Check sheet for the modelled part. Datum: model origin and axes. Units: mm. A direction names the side the tool comes from. Give positions to 0.01 mm unless a question says otherwise; leave off trailing zeros. Order: outer loops, then holes, each group sorted by start corner. A loop starts at its lowest first (then second) coordinate and runs counter-clockwise, first axis right, second up.
Item 1: Sectioned sample at D-D on x = 55.5. Record the boundary of the cut face in (y, z), and give its area (3 significant figures).
Item 2: Release check for a two-part mould opening along Y. For faces 1 (the flat face through (37.99, 15.8, 0.02)), 2 (the cylindrical face through (74.421, 46.854, 0.021)), 3 (the cylindrical face through (0, -20, 0)) record: released by +Y, released by -Y, zero draft, split by the parting line, or undercut.
Item 3: Sectioned sample at B-B on y = 0. Record the boundary of the cut face in (x, z), and give its area (3 significant figures).
Item 4: Sectioned sample at A-A on x = 0. Record the boundary of the cut face in (y, z).
Item 5: Material ranges on line 1 along X through (y, z) = (31.5, -0.2) (3 decimals); line 2 along X through (y, z) = (28.5, -0.85); line 3 along Y through (x, z) = (-65, -0.4) (3 decimals), recorded low to high.
Item 6: Sectioned sample at C-C on z = -1.05. Count the separate pieces of the cut face and the enclosed holes in it, and give its area (3 significant figures).
Item 7: Access from +Z, -Z, +X, -X, +Y, -Y to the whole of each face (thin tool, end or side, straight path). Record for faces 4 (the flat face through (29.325, 29.251, 0.021)), 5 (the flat face through (-1, 17, 1.5)).
Item 8: Gauge pin test, flat end, axial feed: P1, Ø1.5, axis at x = 35, z = 0.5, coming from the -Y side. Record the tip position at first contact, or that the pin passes through.
from build123d import *

# Parameters (mm, degrees)
SKETCH1_R               = 11
SKETCH1_R_2             = 4.075
BOSS_EXTRUDE1_DEPTH     = 1.5
CUT_EXTRUDE1_DEPTH      = 93.138482731
CUT_EXTRUDE1_DEPTH_BACK = 93.138482731
SKETCH2_R               = 1.5
SKETCH3_R               = 1.5
CUT_EXTRUDE2_DEPTH      = 93.138482731
FILLET2_R               = 3


with BuildPart() as part:
    # Sketch1 → Boss-Extrude1 (new, symmetric)
    with BuildSketch(Plane.XY):
        with BuildLine():
            Line((-71.578668004, 35.968657006), (-13.157336008, -15.062685988))
            ThreePointArc((-13.157336008, -15.062685988), (0, -20), (13.157336008, -15.062685988))
            Line((13.157336008, -15.062685988), (71.578668004, 35.968657006))
            ThreePointArc((71.578668004, 35.968657006), (74.362516487, 47.013301158), (65, 53.5))
            Line((65, 53.5), (-65, 53.5))
            ThreePointArc((-65, 53.5), (-74.362516487, 47.013301158), (-71.578668004, 35.968657006))
        make_face()
        Circle(SKETCH1_R, mode=Mode.SUBTRACT)
        with Locations((-65, 43.5)):
            Circle(SKETCH1_R_2, mode=Mode.SUBTRACT)
        with Locations((65, 43.5)):
            Circle(SKETCH1_R_2, mode=Mode.SUBTRACT)
        Polygon((-38.103448276, 45.5), (38.103448276, 45.5), (0, 20), align=None, mode=Mode.SUBTRACT)
        with BuildLine():
            Line((-37.519409883, 34.735340535), (-20.898100342, 23.611848765))
            ThreePointArc((-20.898100342, 23.611848765), (-18.698973233, 12.513928241), (-29.796893758, 10.314801132))
            Line((-29.796893758, 10.314801132), (-46.418203298, 21.438292902))
            ThreePointArc((-46.418203298, 21.438292902), (-48.617330407, 32.536213426), (-37.519409883, 34.735340535))
        make_face(mode=Mode.SUBTRACT)
        with BuildLine():
            Line((37.519409883, 34.735340535), (20.898100342, 23.611848765))
            ThreePointArc((20.898100342, 23.611848765), (18.698973233, 12.513928241), (29.796893758, 10.314801132))
            Line((29.796893758, 10.314801132), (46.418203298, 21.438292902))
            ThreePointArc((46.418203298, 21.438292902), (48.617330407, 32.536213426), (37.519409883, 34.735340535))
        make_face(mode=Mode.SUBTRACT)
    extrude(amount=BOSS_EXTRUDE1_DEPTH, both=True)

    # Sketch2 → Cut-Extrude1 (cut, two sides: drawn at the far end of the back side and taken through both)
    with BuildSketch(Plane.XY.offset(-CUT_EXTRUDE1_DEPTH_BACK)):
        with Locations((0, -15)):
            Circle(SKETCH2_R)
        with Locations((-12.988881057, 7.500866025)):
            Circle(SKETCH2_R)
        with Locations((12.991881057, 7.499133975)):
            Circle(SKETCH2_R)
    extrude(amount=CUT_EXTRUDE1_DEPTH + CUT_EXTRUDE1_DEPTH_BACK, mode=Mode.SUBTRACT)

    # Sketch3 → Cut-Extrude2 (cut, symmetric)
    with BuildSketch(Plane.XY):
        with Locations((-65, 58.5)):
            Circle(SKETCH3_R)
        with Locations((-52.009618943, 36)):
            Circle(SKETCH3_R)
        with Locations((-77.990381057, 36)):
            Circle(SKETCH3_R)
    cut_extrude2 = extrude(amount=CUT_EXTRUDE2_DEPTH, both=True, mode=Mode.SUBTRACT)

    # Mirror1: Cut-Extrude2 across plane
    add(cut_extrude2.mirror(Plane(origin=(0, 0, 0), x_dir=(0, 0, 1), z_dir=(1, 0, 0))), mode=Mode.SUBTRACT)

    # Fillet2
    fillet2_edges = [part.edges().sort_by_distance(p)[0] for p in [
        (0, 20, 0),
        (38.103448276, 45.5, 0),
        (-38.103448276, 45.5, 0),
    ]]
    fillet(fillet2_edges, radius=FILLET2_R)


solid = part.part
Report:
1. outline: (21.92, -1.5) - (53.5, -1.5) - (53.5, 1.5) - (21.92, 1.5) - close
1. area: 94.7 mm2
2. face 1: undercut
2. face 2: split by the parting line
2. face 3: released by -Y
3. outline: (-30.4, -1.5) - (-11, -1.5) - (-11, 1.5) - (-30.4, 1.5) - close; (11, -1.5) - (30.4, -1.5) - (30.4, 1.5) - (11, 1.5) - close
3. area: 116 mm2
4. outline: (-20, -1.5) - (-16.5, -1.5) - (-16.5, 1.5) - (-20, 1.5) - close; (-13.5, -1.5) - (-11, -1.5) - (-11, 1.5) - (-13.5, 1.5) - close; (11, -1.5) - (20.61, -1.5) - (20.61, 1.5) - (11, 1.5) - close; (45.5, -1.5) - (53.5, -1.5) - (53.5, 1.5) - (45.5, 1.5) - close
5. line 1: x = -66.463 to -49.204, -32.685 to -17.184, 17.184 to 32.685, 49.204 to 66.463
5. line 2: x = -63.03 to -49.96, -28.2 to -12.7, 12.7 to 28.2, 49.96 to 63.03
5. line 3: y = 30.222 to 39.425, 47.575 to 53.5
6. separate pieces: 1
6. enclosed holes: 11
6. area: 4,490 mm2
7. face 4: +Z, -Z
7. face 5: +Z, +X, -X, +Y, -Y
8. P1: stops at y = 3.36
